Part model, mm, in its own coordinate system. Face numbers are marked on the shaded views. A direction names the side the tool comes from. Give positions to 0.01 mm unless a question says otherwise; leave off trailing zeros. Loops run counter-clockwise (first coordinate to the right, second up) from the corner with the lowest first, then second, coordinate; pieces in that order, holes last. Notation, with made-up numbers: M -3.5,49.5 L 44.5,49.5 A25 cw 44.5,79.5 Z; hole C 82,-37.5 d4. An arc over 180 degrees is marked long. Answer in a Markdown table with one row per item.
from build123d import *

# Parameters (mm, degrees)
BOSS_EXTRUDE1_DEPTH = 36
SKETCH4_R           = 1.05
SKETCH4_W           = 8.5
SKETCH4_H           = 8.5
CUT_EXTRUDE1_DEPTH  = 86.201472175
SKETCH4_3_W         = 27.5
SKETCH4_3_H         = 26.5
SKETCH4_3_W_2       = 25
SKETCH4_3_H_2       = 24
SKETCH4_3_R         = 1.05
SKETCH4_3_W_3       = 8.5
SKETCH4_3_H_3       = 8.5
CUT_EXTRUDE2_DEPTH  = 1.7
SKETCH5_W           = 17
SKETCH5_H           = 20
CUT_EXTRUDE3_DEPTH  = 1.7
FILLET1_R           = 0.5
BOSS_EXTRUDE2_DEPTH = 1
FILLET2_R           = 1
FILLET3_R           = 1


with BuildPart() as part:
    # Sketch2 → Boss-Extrude1 (new body)
    with BuildSketch(Plane.XY):
        with BuildLine():
            Line((0, 0), (-25.184422383, 51.63571796))
            Line((-25.184422383, 51.63571796), (-48.384422383, 51.63571796))
            ThreePointArc((-48.384422383, 51.63571796), (-49.378944278, 52.531189497), (-48.592334074, 53.613865561))
            Line((-48.592334074, 53.613865561), (-25.654772837, 58.48939471))
            Line((-25.654772837, 58.48939471), (-0.392745057, 6.694562109))
            ThreePointArc((-0.392745057, 6.694562109), (1.056036581, 0.865561175), (0, -5.047222168))
            Line((0, -5.047222168), (-23.13, -5.047222168))
            ThreePointArc((-23.13, -5.047222168), (-23.667026027, -4.875521503), (-24.040049398, -4.452754858))
            Line((-24.040049398, -4.452754858), (-24.527781987, -3.452754858))
            ThreePointArc((-24.527781987, -3.452754858), (-24.476528577, -2.474781543), (-23.62, -2))
            Line((-23.62, -2), (0, -2))
            Line((0, -2), (0, 0))
        make_face()
    extrude(amount=BOSS_EXTRUDE1_DEPTH)

    # Sketch4 → Cut-Extrude1 (cut, through all)
    with BuildSketch(Plane(origin=(2.320421937, 1.131745398, 0), x_dir=(0, 0, -1), z_dir=(0.898794046299168, 0.4383711467890754, 0))):
        with Locations(Location((-28.5, 51.816231926, 0), (0, 0, 90))):
            Circle(SKETCH4_R)
        with Locations(Location((-28.5, 39.316231926, 0), (0, 0, 90))):
            Circle(SKETCH4_R)
        with Locations(Location((-7.5, 51.816231926, 0), (0, 0, 90))):
            Circle(SKETCH4_R)
        with Locations(Location((-7.5, 39.316231926, 0), (0, 0, 90))):
            Circle(SKETCH4_R)
        with Locations((-18, 39.316231926)):
            Rectangle(SKETCH4_W, SKETCH4_H)
    extrude(amount=-CUT_EXTRUDE1_DEPTH, mode=Mode.SUBTRACT)

    # Sketch4<3> → Cut-Extrude2 (cut)
    # profile 1 of 2: a face of its own
    with BuildSketch(Plane(origin=(2.320421937, 1.131745398, 0), x_dir=(0, 0, -1), z_dir=(0.898794046299168, 0.4383711467890754, 0))):
        with Locations((-18, 41.816231926)):
            Rectangle(SKETCH4_3_W, SKETCH4_3_H)
        with Locations((-18, 41.816231926)):
            Rectangle(SKETCH4_3_W_2, SKETCH4_3_H_2, mode=Mode.SUBTRACT)
    # profile 2 of 2: a face of its own
    with BuildSketch(Plane(origin=(2.320421937, 1.131745398, 0), x_dir=(0, 0, -1), z_dir=(0.898794046299168, 0.4383711467890754, 0))):
        with Locations((-18, 41.816231926)):
            Rectangle(SKETCH4_3_W_2, SKETCH4_3_H_2)
        with Locations(Location((-7.5, 39.316231926, 0), (0, 0, 90))):
            Circle(SKETCH4_3_R, mode=Mode.SUBTRACT)
        with Locations(Location((-7.5, 51.816231926, 0), (0, 0, 90))):
            Circle(SKETCH4_3_R, mode=Mode.SUBTRACT)
        with Locations(Location((-28.5, 39.316231926, 0), (0, 0, 90))):
            Circle(SKETCH4_3_R, mode=Mode.SUBTRACT)
        with Locations(Location((-28.5, 51.816231926, 0), (0, 0, 90))):
            Circle(SKETCH4_3_R, mode=Mode.SUBTRACT)
        with Locations((-18, 39.316231926)):
            Rectangle(SKETCH4_3_W_3, SKETCH4_3_H_3, mode=Mode.SUBTRACT)
    extrude(amount=-CUT_EXTRUDE2_DEPTH, mode=Mode.SUBTRACT)

    # Sketch5 → Cut-Extrude3 (cut)
    with BuildSketch(Plane(origin=(2.320421937, 1.131745398, 0), x_dir=(0, 0, -1), z_dir=(0.898794046299168, 0.4383711467890754, 0))):
        with Locations((-18, 19.816231926)):
            Rectangle(SKETCH5_W, SKETCH5_H)
    extrude(amount=-CUT_EXTRUDE3_DEPTH, mode=Mode.SUBTRACT)

    # Fillet1
    fillet1_edges = [part.edges().sort_by_distance(p)[0] for p in [
        (0, 0, 18),
        (-25.184422383, 51.63571796, 18),
    ]]
    fillet(fillet1_edges, radius=FILLET1_R)

    # Sketch6 → Boss-Extrude2 (add)
    with BuildSketch(Plane.XY.offset(36)):
        with BuildLine():
            Line((-0.392745057, 6.694562109), (-3.392745057, 6.694562109))
            ThreePointArc((-3.392745057, 6.694562109), (-4.80695862, 6.108775671), (-5.392745057, 4.694562109))
            Line((-5.392745057, 4.694562109), (-5.392745057, -5.047222168))
            Line((-5.392745057, -5.047222168), (0, -5.047222168))
            ThreePointArc((0, -5.047222168), (1.056036581, 0.865561175), (-0.392745057, 6.694562109))
        make_face()
    boss_extrude2 = extrude(amount=BOSS_EXTRUDE2_DEPTH)

    # Fillet2
    # the kernel refuses this fillet: 1 mm, written as the material it adds along each edge
    with BuildSketch(Plane(origin=(-5.392745057, -2, 36), x_dir=(-1, 0, 0), z_dir=(0, -1, 0))) as fillet2_piece_1:
        with BuildLine():
            CenterArc((FILLET2_R, -FILLET2_R), FILLET2_R, 90, 90)
            Line((0, -FILLET2_R), (0, 0))
            Line((0, 0), (FILLET2_R, 0))
        make_face()
    extrude(amount=3.047222168)
    with BuildSketch(Plane(origin=(2.107254943, 6.694562109, 36), x_dir=(0, 0, 1), z_dir=(-1, 0, 0))) as fillet2_piece_2_section:
        with BuildLine():
            CenterArc((FILLET2_R, FILLET2_R), FILLET2_R, 180, 90)
            Line((0, FILLET2_R), (0, 0))
            Line((0, 0), (FILLET2_R, 0))
        make_face()
    fillet2_piece_2 = extrude(amount=7.872411049, mode=Mode.PRIVATE)
    fillet2_piece_2 = split(fillet2_piece_2, bisect_by=Plane(origin=(-0.632231225, 7.185581517, 36.086380113), z_dir=(-0.8987940462991679, -0.4383711467890754, 0)), keep=Keep.TOP, mode=Mode.PRIVATE)
    fillet2_piece_2 = split(fillet2_piece_2, bisect_by=Plane(origin=(-2.952653161, 6.053836119, 36.086380113), z_dir=(0.898794046299168, 0.43837114678907535, 0)), keep=Keep.TOP, mode=Mode.PRIVATE)
    add(fillet2_piece_2)

    # Mirror3: Boss-Extrude2 across plane
    add(boss_extrude2.mirror(Plane(origin=(0, 0, 18), x_dir=(1, 0, 0), z_dir=(0, 0, -1))))

    # Fillet3
    # the kernel refuses this fillet: 1 mm, written as the material it adds along each edge
    with BuildSketch(Plane(origin=(-5.392745057, -2, 0), x_dir=(-1, 0, 0), z_dir=(0, -1, 0))) as fillet3_piece_1:
        with BuildLine():
            CenterArc((FILLET3_R, FILLET3_R), FILLET3_R, 180, 90)
            Line((0, FILLET3_R), (0, 0))
            Line((0, 0), (FILLET3_R, 0))
        make_face()
    extrude(amount=3.047222168)
    with BuildSketch(Plane(origin=(2.107254943, 6.694562109, 0), x_dir=(0, 1, 0), z_dir=(-1, 0, 0))) as fillet3_piece_2_section:
        with BuildLine():
            CenterArc((FILLET3_R, FILLET3_R), FILLET3_R, 180, 90)
            Line((0, FILLET3_R), (0, 0))
            Line((0, 0), (FILLET3_R, 0))
        make_face()
    fillet3_piece_2 = extrude(amount=7.872411049, mode=Mode.PRIVATE)
    fillet3_piece_2 = split(fillet3_piece_2, bisect_by=Plane(origin=(-2.952649492, 6.053828597, -0.086392955), z_dir=(0.8987940462991654, 0.43837114678908073, 0)), keep=Keep.TOP, mode=Mode.PRIVATE)
    fillet3_piece_2 = split(fillet3_piece_2, bisect_by=Plane(origin=(-0.632227556, 7.185573995, -0.086392955), z_dir=(-0.8987940462991654, -0.43837114678908073, 0)), keep=Keep.TOP, mode=Mode.PRIVATE)
    add(fillet3_piece_2)


solid = part.part
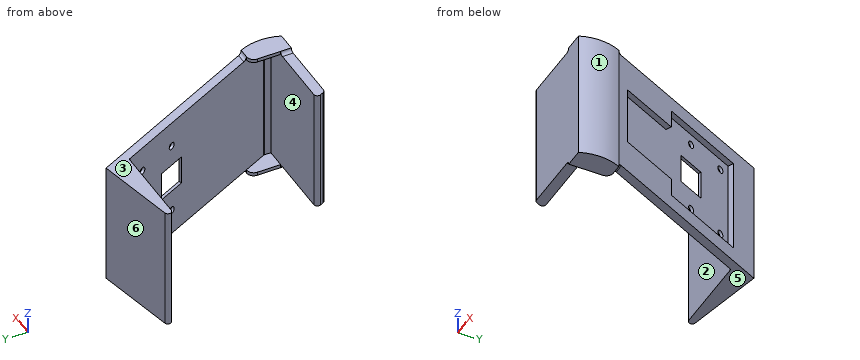
(1) Saw through at B-B (z = 19.5). Write the cut outline in (x, y), plus the area to 3 significant figures.
Recorded:
| item | result |
|---|---|
| outline | M -48.59,53.61 A1 ccw -48.38,51.64 L -25.5,51.64 A0.5 cw -25.05,51.35 L -19.1,39.16 L -18.31,39.54 L -23.35,49.88 L -21.82,50.62 L -25.65,58.49 Z; M -24.53,-3.45 L -24.04,-4.45 A1.06 ccw -23.13,-5.05 L 0,-5.05 A14.39 ccw -0.39,6.69 L -1.98,9.95 L -3.51,9.21 L -14.58,31.9 L -15.37,31.52 L -0.05,0.1 A0.5 cw 0,-0.12 L 0,-2 L -23.62,-2 A1.01 ccw Z |
| area | 251 mm^2 |
(2) Saw through at D-D (y = 17.5). Write the cut outline in (x, z), plus the area to 3 significant figures.
Recorded:
| item | result |
|---|---|
| outline | M -8.54,0 L -5.66,0 L -5.66,9.5 L -7.55,9.5 L -7.55,26.5 L -5.66,26.5 L -5.66,36 L -8.54,36 Z |
| area | 71.3 mm^2 |
(3) Saw through at C-C (x = -11). Write the cut outline in (y, z), plus the area to 3 significant figures.
Recorded:
| item | result |
|---|---|
| outline | M -5.05,0 L -2,0 L -2,36 L -5.05,36 Z; M 22.55,0 L 28.44,0 L 28.44,4.25 L 26.42,4.25 L 26.42,9.5 L 24.56,9.5 L 24.56,26.5 L 26.42,26.5 L 26.42,31.75 L 28.44,31.75 L 28.44,36 L 22.55,36 Z |
| area | 235 mm^2 |
(4) Drill centre lines: line 1 along Y through (x, z) = (-22.5, 8); line 2 along Y through (x, z) = (-23, 30); line 3 along Y through (x, z) = (-17, 21). Where is each one in solid material? Low to high.
Recorded:
| item | result |
|---|---|
| line 1 | y = -5.05 to -2, 47.7 to 48.14, 50.29 to 52.02 |
| line 2 | y = -5.05 to -2, 47.16 to 49.17, 50.05 to 53.05 |
| line 3 | y = -5.05 to -2 |
(5) Pin check, flat tips, straight feed: pin 1 Ø8 at (y, z) = (38, 32) entering from -X; pin 2 Ø24.5 at (x, y) = (-28.5, 24) entering from -Z; pin 3 Ø14.5 at (x, y) = (-20, 44) entering from +Z; pin 4 Ø6 at (y, z) = (44, 27.5) entering from -X. Stop position of each tip, or through.
Recorded:
| item | result |
|---|---|
| pin 1 | stops at x = -20.48 |
| pin 2 | passes through |
| pin 3 | stops at z = 36 |
| pin 4 | stops at x = -22.92 |
(6) Pull direction Z, two halves, no side cores. Call the marked faces 3, 4, 5 and 6: +Z half, -Z half, draft (parallel to the pull), parting line (faces both ways), or undercut.
Recorded:
| item | result |
|---|---|
| face 3 | +Z half |
| face 4 | undercut |
| face 5 | -Z half |
| face 6 | draft |
(7) Which spindle directions (+Z, -Z, +X, -X, +Y, -Y) get a long thin tool onto all of the face, cutting with end or side? Do the marked faces 1 and 2. Say none if no direction does.
Recorded:
| item | result |
|---|---|
| face 1 | +Z, -Z, +X |
| face 2 | +Z, -Z, -X, -Y |
(8) Saw through at A-A (z = 12). Write the cut outline in (x, y).
Recorded:
| item | result |
|---|---|
| outline | M -48.59,53.61 A1 ccw -48.38,51.64 L -25.5,51.64 A0.5 cw -25.05,51.35 L -0.05,0.1 A0.5 cw 0,-0.12 L 0,-2 L -23.62,-2 A1.01 ccw -24.53,-3.45 L -24.04,-4.45 A1.06 ccw -23.13,-5.05 L 0,-5.05 A14.39 ccw -0.39,6.69 L -1.98,9.95 L -3.51,9.21 L -23.35,49.88 L -21.82,50.62 L -25.65,58.49 Z |
